Verification items for the finished model (mm, model axes). A direction names the side the tool comes from. Give positions to 0.01 mm unless a question says otherwise; leave off trailing zeros. Loops run counter-clockwise (first coordinate to the right, second up) from the corner with the lowest first, then second, coordinate; pieces in that order, holes last. Notation, with made-up numbers: (31, -7) - (51, -7) arc R29 cw to (51, 23) - close; hole circle Ø8 at (-26, 21.25). An arc over 180 degrees is marked (long way). One line per item, written item: value. Start each with the question number.
1. Sectioned sample at C-C (x = 0). Record the cut outline in (y, z).
2. Sectioned sample at A-A (y = 1.25). Record the cut outline in (x, z), plus the area to 3 significant figures.
3. Gauge pin test, flat ends, axial feed: pin 1 (3 mm diameter, centred on x = -0.5, z = -33.5, fed in from +Y); pin 2 (1.5 mm diameter, centred on y = 3.5, z = -18.5, fed in from -X); pin 3 (3 mm diameter, centred on x = 2, y = -1, fed in from +Z). Record the tip position at first contact, or that the pin passes through.
4. Access from +Z, -Z, +X, -X, +Y, -Y to the whole of each face (thin tool, end or side, straight path). Record for faces 1 (the cylindrical face through (-1.08, -4.88, -0.99)), 2 (the cylindrical face through (-1.867, 3.905, 9.367)), 3 (the cylindrical face through (-3, 0, -27)).
5. Scan lines: L1, parallel to Z at x = 4, y = -0.5; L2, parallel to X at y = 0.25, z = -45; L3, parallel to X at y = -2.5, z = 15.5. Record each from-to range of solid material in increasing order. Write a range as [from, to].
6. Sectioned sample at D-D (z = 16). Record the cut outline in (x, y).
7. Sectioned sample at B-B (z = -47). Record the cut outline in (x, y).
Autodesk Inventor part; units mm, degrees
ref_plane "YZ Plane" through (0, 0, 0) normal (1, 0, 0) x (0, 1, 0)
ref_plane "XZ Plane" through (0, 0, 0) normal (0, 1, 0) x (-1, 0, 0)
ref_plane "XY Plane" through (0, 0, 0) normal (0, 0, 1) x (1, 0, 0)
sketch "Sketch1" plane through (0, 0, 0) normal (0, 0, 1) x (1, 0, 0)
  circle A0 centre (0, 0) radius 6
  circle A1 centre (0, 0) radius 5
  point P0 (0, 0)
  dimension "d0" = 1
extrude "Extrusion1" add sketch "Sketch1" against normal blind 2 contours A1
sketch "Sketch2" plane through (0, 0, -2) normal (0, 0, 1) x (1, 0, 0)
  circle A0 centre (0, 0) radius 3
  circle A1 centre (0, 0) radius 5
  point P0 (0, 0)
extrude "Extrusion2" add sketch "Sketch2" against normal blind 50 contours A0
sketch "Sketch3" plane through (0, 0, 0) normal (0, 0, 1) x (1, 0, 0)
  circle A0 centre (-1, 0) radius 4
  circle A1 centre (0, 0) radius 5
  point P0 (0, 0)
  dimension "d9" = 8
extrude "Extrusion3" add sketch "Sketch3" along normal blind 23 contours A0
fillet "Fillet2" radius 4 1 edges at (-5, 0, 23)
properties part number "handle_base_rod"
Results are:
1. outline: (-5, -2) - (-3, -2) - (-3, -52) - (3, -52) - (3, -2) - (5, -2) - (5, 0) - (3.87, 0) - (3.87, 19) arc R3.87 ccw to (-3.87, 19) - (-3.87, 0) - (-5, 0) - close
2. outline: (-4.84, -2) - (-2.73, -2) - (-2.73, -52) - (2.73, -52) - (2.73, -2) - (4.84, -2) - (4.84, 0) - (2.8, 0) - (2.8, 19) arc R3.8 ccw to (-4.8, 19) - (-4.8, 0) - (-4.84, 0) - close
2. area: 459 mm^2
3. pin 1: stops at y = 3
3. pin 2: stops at x = -1.2
3. pin 3: stops at z = 22.64
4. face 1: +Z, -Z
4. face 2: +Z
4. face 3: -Z
5. L1: z = [-2, 0]
5. L2: x = [-2.99, 2.99]
5. L3: x = [-4.12, 2.12]
6. outline: circle Ø8 at (-1, 0)
7. outline: circle Ø6 at (0, 0)
